```python
from build123d import *

# Parameters (mm, degrees)
SKETCH2_W           = 80.01
SKETCH2_H           = 36.195
BOSS_EXTRUDE1_DEPTH = 1.6002
SKETCH3_W           = 71.12
SKETCH3_H           = 24.0792
BOSS_EXTRUDE2_DEPTH = 7.239
SKETCH4_R           = 1.4605
CUT_EXTRUDE1_DEPTH  = 1.6002
BOSS_EXTRUDE3_DEPTH = 2.54
SKETCH6_W           = 50.8
SKETCH6_H           = 6.0325
SKETCH6_H_2         = 13.7795
BOSS_EXTRUDE5_DEPTH = 2.54
SKETCH9_W           = 50.8
SKETCH9_H           = 19.812
BOSS_EXTRUDE6_DEPTH = 8.89


with BuildPart() as part:
    # Sketch2 → Boss-Extrude1 (new body)
    with BuildSketch(Plane.XY):
        Rectangle(SKETCH2_W, SKETCH2_H)
    extrude(amount=BOSS_EXTRUDE1_DEPTH)

    # Sketch3 → Boss-Extrude2 (add)
    with BuildSketch(Plane.XY.offset(1.6002)):
        Rectangle(SKETCH3_W, SKETCH3_H)
    extrude(amount=BOSS_EXTRUDE2_DEPTH)

    # Sketch4 → Cut-Extrude1 (cut)
    with BuildSketch(Plane.XY.offset(1.6002)):
        with Locations((-37.5285, 15.621)):
            Circle(SKETCH4_R)
        with Locations(Location((37.5285, 15.621, 0), (0, 0, 180))):
            Circle(SKETCH4_R)
        with Locations((37.5285, -15.621)):
            Circle(SKETCH4_R)
        with Locations(Location((-37.5285, -15.621, 0), (0, 0, 180))):
            Circle(SKETCH4_R)
    extrude(amount=-CUT_EXTRUDE1_DEPTH, mode=Mode.SUBTRACT)

    # Sketch5 → Boss-Extrude3 (add)
    with BuildSketch(Plane.XY.offset(1.6002)):
        Polygon((35.56, 6.223), (39.624, 2.159), (39.624, -2.159), (35.56, -6.223), align=None)
    extrude(amount=BOSS_EXTRUDE3_DEPTH)

    # Sketch6 → Boss-Extrude5 (add)
    with BuildSketch(Plane(origin=(0, 0, 0), x_dir=(-1, 0, 0), z_dir=(0, 0, -1))):
        with Locations((10.16, 15.08125)):
            Rectangle(SKETCH6_W, SKETCH6_H)
        with Locations((10.16, 5.17525)):
            Rectangle(SKETCH6_W, SKETCH6_H_2)
        Polygon((-15.24, 12.065), (-35.56, 12.065), (-35.56, -12.065), (35.56, -12.065), (35.56, -1.7145), (-15.24, -1.7145), align=None)
    extrude(amount=BOSS_EXTRUDE5_DEPTH)

    # Sketch9 → Boss-Extrude6 (add)
    with BuildSketch(Plane(origin=(0, 0, -2.54), x_dir=(-1, 0, 0), z_dir=(0, 0, -1))):
        with Locations((10.16, 8.1915)):
            Rectangle(SKETCH9_W, SKETCH9_H)
    extrude(amount=BOSS_EXTRUDE6_DEPTH)


solid = part.part
```
Work out the finished part from the listing and answer in its coordinate system (mm). A direction names the side the tool comes from. Coordinates: 2 decimals unless noted, no trailing zeros. Loops run counter-clockwise (first coordinate to the right, second up) from the corner with the lowest first, then second, coordinate; pieces in that order, holes last. Notation, with made-up numbers: (-13, 59.25) - (38, 59.25) arc R20 cw to (38, 90.25) - close; hole circle Ø10 at (42, 73). An arc over 180 degrees is marked (long way). Use a Markdown table: item, result.
Item 1: Find section A-A, the plane z = 3.25. Determine the outline of the cut face in (x, y), and give its area (3 significant figures).
Evaluation:
| item | result |
|---|---|
| outline | (-35.56, -12.04) - (35.56, -12.04) - (35.56, -6.22) - (39.62, -2.16) - (39.62, 2.16) - (35.56, 6.22) - (35.56, 12.04) - (-35.56, 12.04) - close |
| area | 1,750 mm2 |
Item 2: For faces 4 (the flat face through (37, 0, 4.14)), 5 (the flat face through (-35.56, 0, 5)), 6 (the flat face through (-10, -1.715, -7)), 7 (the flat face through (35.56, 0, -1)), 8 (the flat face through (25, 12.065, -1)), determine the directions among +Z, -Z, +X, -X, +Y, -Y from which every point of the face is accessible in a straight line to the end or side of a thin tool.
Evaluation:
| item | result |
|---|---|
| face 4 | +Z, +X, +Y, -Y |
| face 5 | +Z, -X, +Y, -Y |
| face 6 | -Z, +X, -X, -Y |
| face 7 | -Z, +X, +Y, -Y |
| face 8 | -Z, +X, +Y |
Item 3: The mould has two halves that part along X. Classify faces 1 (the cylindrical face through (-36.37, -14.73, 0.81)), 2 (the flat face through (37.564, 4.219, 2.852)), 3 (the flat face through (0, 12.04, 5)): +X half, -X half, draft (parallel to the pull), parting line (faces both ways), or undercut.
Evaluation:
| item | result |
|---|---|
| face 1 | undercut |
| face 2 | +X half |
| face 3 | draft |
Item 4: Consider probe 1 along Y at (x, z) = (34.5, -1) (3 decimals); probe 2 along Z at (x, y) = (27.5, 5.5); probe 3 along Y at (x, z) = (19, 4). Determine where each line is inside the solid, lowest interval first. Write a range as from..to.
Evaluation:
| item | result |
|---|---|
| probe 1 | y = -12.065..12.065 |
| probe 2 | z = -2.54..8.84 |
| probe 3 | y = -12.04..12.04 |
Item 5: Given pin 1 Ø1.3 at (x, z) = (24, -1) entering from +Y (3 decimals); pin 2 Ø3 at (y, z) = (2, -0.5) entering from -X (3 decimals); pin 3 Ø9 at (y, z) = (10.5, -6) entering from +X; pin 4 Ø3.5 at (y, z) = (-2.5, 5) entering from +X, each flat-ended and moving along its own axis, determine where each tip first touches the part or whether it passes through.
Evaluation:
| item | result |
|---|---|
| pin 1 | stops at y = 12.065 |
| pin 2 | stops at x = -40.005 |
| pin 3 | stops at x = 35.56 |
| pin 4 | stops at x = 39.62 |
Item 6: Find section C-C, the plane x = 26.5. Determine the outline of the cut face in (y, z) (1 decimal).
Evaluation:
| item | result |
|---|---|
| outline | (-18.1, 0) - (-12.1, 0) - (-12.1, -2.5) - (12.1, -2.5) - (12.1, 0) - (18.1, 0) - (18.1, 1.6) - (12, 1.6) - (12, 8.8) - (-12, 8.8) - (-12, 1.6) - (-18.1, 1.6) - close |
Item 7: Find section B-B, the plane y = -10. Determine the outline of the cut face in (x, z) (3 decimals).
Evaluation:
| item | result |
|---|---|
| outline | (-40.005, 0) - (-35.56, 0) - (-35.56, -2.54) - (35.56, -2.54) - (35.56, 0) - (40.005, 0) - (40.005, 1.6) - (35.56, 1.6) - (35.56, 8.839) - (-35.56, 8.839) - (-35.56, 1.6) - (-40.005, 1.6) - close |
Item 8: Find section D-D, the plane z = -7. Determine the outline of the cut face in (x, y).
Evaluation:
| item | result |
|---|---|
| outline | (-35.56, -1.71) - (15.24, -1.71) - (15.24, 18.1) - (-35.56, 18.1) - close |
